Part model, mm, in its own coordinate system. A direction names the side the tool comes from. Give positions to 0.01 mm unless a question says otherwise; leave off trailing zeros. Order: outer loops, then holes, each group sorted by start corner. A loop starts at its lowest first (then second) coordinate and runs counter-clockwise, first axis right, second up. Notation, with made-up numbers: M -39,8.25 L -22,8.25 A3 cw -22,12.25 Z; hole C 23,65.5 d5. An arc over 180 degrees is marked long. Answer as a JSON object with one key per item and string values.
from build123d import *

# Parameters (mm, degrees)
SALIENTE_EXTRUIR1_DEPTH = 1.5
CROQUIS9_W              = 48.051342352
CROQUIS9_H              = 38
SALIENTE_EXTRUIR7_DEPTH = 2
CROQUIS10_W             = 8
CROQUIS10_H             = 1.5
SALIENTE_EXTRUIR8_DEPTH = 5
REDONDEO1_R             = 2
REVOLUCI_N1_ANGLE       = 180
CROQUIS14_R             = 11.15
CROQUIS14_R_2           = 10.15
SALIENTE_EXTRUIR9_DEPTH = 2.5
CORTAR_EXTRUIR4_DEPTH   = 2.5


with BuildPart() as part:
    # Croquis1 → Saliente-Extruir1 (new body)
    with BuildSketch(Plane(origin=(0, 0, 0), x_dir=(1, 0, 0), z_dir=(0, 1, 0))):
        with BuildLine():
            Line((-25.5, -22.5), (25.5, -22.5))
            ThreePointArc((25.5, -22.5), (26.914213562, -21.914213562), (27.5, -20.5))
            Line((27.5, -20.5), (27.5, 20.5))
            ThreePointArc((27.5, 20.5), (26.914213562, 21.914213562), (25.5, 22.5))
            Line((25.5, 22.5), (-25.5, 22.5))
            ThreePointArc((-25.5, 22.5), (-26.914213562, 21.914213562), (-27.5, 20.5))
            Line((-27.5, 20.5), (-27.5, -20.5))
            ThreePointArc((-27.5, -20.5), (-26.914213562, -21.914213562), (-25.5, -22.5))
        make_face()
    extrude(amount=SALIENTE_EXTRUIR1_DEPTH)

    # Croquis9 → Saliente-Extruir7 (add)
    with BuildSketch(Plane(origin=(0, 1.5, 0), x_dir=(1, 0, 0), z_dir=(0, 1, 0))):
        with BuildLine():
            Line((-24.243818065, 20.5), (24.192475714, 20.5))
            ThreePointArc((24.192475714, 20.5), (25.117035003, 20.117035003), (25.5, 19.192475714))
            Line((25.5, 19.192475714), (25.5, -19.192475714))
            ThreePointArc((25.5, -19.192475714), (25.117035003, -20.117035003), (24.192475714, -20.5))
            Line((24.192475714, -20.5), (-24.243818065, -20.5))
            ThreePointArc((-24.243818065, -20.5), (-25.168377355, -20.117035003), (-25.551342352, -19.192475714))
            Line((-25.551342352, -19.192475714), (-25.551342352, 19.192475714))
            ThreePointArc((-25.551342352, 19.192475714), (-25.168377355, 20.117035003), (-24.243818065, 20.5))
        make_face()
        with Locations((-0.025671176, 0)):
            Rectangle(CROQUIS9_W, CROQUIS9_H, mode=Mode.SUBTRACT)
    extrude(amount=SALIENTE_EXTRUIR7_DEPTH)

    # Croquis10 → Saliente-Extruir8 (add)
    with BuildSketch(Plane(origin=(0, 3.5, 0), x_dir=(1, 0, 0), z_dir=(0, 1, 0))):
        with Locations((0, 19.75)):
            Rectangle(CROQUIS10_W, CROQUIS10_H)
        with Locations((0, -19.75)):
            Rectangle(CROQUIS10_W, CROQUIS10_H)
    extrude(amount=SALIENTE_EXTRUIR8_DEPTH)

    # Redondeo1
    redondeo1_edges = [part.edges().sort_by_distance(p)[0] for p in [
        (-4, 8.5, -19.75),
        (4, 8.5, -19.75),
        (4, 8.5, 19.75),
        (-4, 8.5, 19.75),
    ]]
    fillet(redondeo1_edges, radius=REDONDEO1_R)

    # Croquis13 → Revolución1 (revolve)
    with BuildSketch(Plane.XY.offset(20.5)):
        with BuildLine():
            Line((0, 7.25), (0, 4.75))
            ThreePointArc((0, 4.75), (-1.25, 6), (0, 7.25))
        make_face()
    revoluci_n1 = revolve(axis=Axis((0, -1000, 20.5), (0, 1, 0)), revolution_arc=REVOLUCI_N1_ANGLE)

    # Simetría1: Revolución1 across plane
    add(revoluci_n1.mirror(Plane.XY))

    # Croquis14 → Saliente-Extruir9 (add)
    # profile 1 of 2: a face of its own
    with BuildSketch(Plane(origin=(0, 1.5, 0), x_dir=(1, 0, 0), z_dir=(0, 1, 0))):
        with Locations(Location((11.998657648, -7, 0), (0, 0, 270))):
            Circle(CROQUIS14_R)
        with Locations(Location((11.998657648, -7, 0), (0, 0, 270))):
            Circle(CROQUIS14_R_2, mode=Mode.SUBTRACT)
    # profile 2 of 2: a face of its own
    with BuildSketch(Plane(origin=(0, 1.5, 0), x_dir=(1, 0, 0), z_dir=(0, 1, 0))):
        with Locations(Location((-12.05, 7, 0), (0, 0, 270))):
            Circle(CROQUIS14_R)
        with Locations(Location((-12.05, 7, 0), (0, 0, 270))):
            Circle(CROQUIS14_R_2, mode=Mode.SUBTRACT)
    extrude(amount=SALIENTE_EXTRUIR9_DEPTH)

    # Croquis15 → Cortar-Extruir4 (cut)
    with BuildSketch(Plane(origin=(0, 1.5, 0), x_dir=(1, 0, 0), z_dir=(0, 1, 0))):
        Polygon((-12.553109789, 6.135777494), (11.495547859, -7.864222506), (12.501767438, -6.135777494), (-11.546890211, 7.864222506), align=None)
    extrude(amount=CORTAR_EXTRUIR4_DEPTH, mode=Mode.SUBTRACT)


solid = part.part
1. Two-plate mould, pull along Z, no slides. Class faces 1 (the cylindrical face through (-3.43, 7.9, -19.76)), 2 (the cylindrical face through (-21.438, 2.732, -13.016)), 3 (the cylindrical face through (-25.178, 2.486, -20.107)): +Z half, -Z half, draft (parallel to the pull), parting line (faces both ways), or undercut.
Worked answers:
{"face 1": "draft", "face 2": "undercut", "face 3": "-Z half"}
2. Pin check, flat tips, straight feed: P1, Ø1.5, axis at y = 4.5, z = -10, coming from the +X side; P2, Ø3.5, axis at x = 12, y = 6.5, coming from the +Z side; P3, Ø3, axis at x = 2.5, y = 4, coming from the -Z side; P4, Ø19, axis at x = -7.5, z = -6, coming from the +Y side. Stop position of each tip, or through.
Worked answers:
{"P1": "stops at x = -1.17", "P2": "passes through", "P3": "stops at z = -20.5", "P4": "stops at y = 4"}
3. Cut at A-A on z = 7. Give the cut face in (x, y).
Worked answers:
{"outline": "M -27.5,0 L 27.5,0 L 27.5,1.5 L 25.5,1.5 L 25.5,3.5 L 24,3.5 L 24,1.5 L 23.15,1.5 L 23.15,4 L 22.15,4 L 22.15,1.5 L 1.85,1.5 L 1.85,4 L 0.85,4 L 0.85,1.5 L -24.05,1.5 L -24.05,3.5 L -25.55,3.5 L -25.55,1.5 L -27.5,1.5 Z"}
4. Which spindle directions (+Z, -Z, +X, -X, +Y, -Y) get a long thin tool onto all of the face, cutting with end or side? Do faces 4 (the flat face through (15, 4, 17)), 5 (the flat face through (0, 3, -19)), 6 (the cylindrical face through (25.127, 2.486, 20.107)). Say none if no direction does.
Worked answers:
{"face 4": "+X, -X, +Y", "face 5": "+Y", "face 6": "+Z, +X, +Y"}
5. Cut at B-B on x = -12.05. Give the cut face in (y, z), plus the area to 3 significant figures.
Worked answers:
{"outline": "M 0,-22.5 L 1.5,-22.5 L 1.5,-20.5 L 3.5,-20.5 L 3.5,-19 L 1.5,-19 L 1.5,-18.15 L 4,-18.15 L 4,-17.15 L 1.5,-17.15 L 1.5,3.15 L 4,3.15 L 4,4.15 L 1.5,4.15 L 1.5,19 L 3.5,19 L 3.5,20.5 L 1.5,20.5 L 1.5,22.5 L 0,22.5 Z", "area": "78.5 mm^2"}
6. Probe line 1 along X through (y, z) = (3.15, -7); line 2 along Z through (x, y) = (-12.05, 2.85); line 3 along X through (y, z) = (2.9, 7). List the from-to ranges inside material, lowest first.
Worked answers:
{"line 1": "x = -25.55 to -24.05, -23.2 to -22.2, -1.9 to -0.9, 24 to 25.5", "line 2": "z = -20.5 to -19, -18.15 to -17.15, 3.15 to 4.15, 19 to 20.5", "line 3": "x = -25.55 to -24.05, 0.85 to 1.85, 22.15 to 23.15, 24 to 25.5"}
